Here's the drawing with two shaded views (mm, measured from the low corner). I have some questions. A direction names the side the tool comes from. Round coordinates to 2 decimals unless told otherwise and drop trailing zeros. Order: outer loops, then holes, each group sorted by start corner. A loop starts at its lowest first (then second) coordinate and runs counter-clockwise, first axis right, second up. Notation, with made-up numbers: (82, 20) -> (97, 20) arc R23 cw to (97, 35) -> close; hole circle Ø8 at (-25, 68). An arc over 180 degrees is marked (long way). Answer in a Markdown table with one row per item.
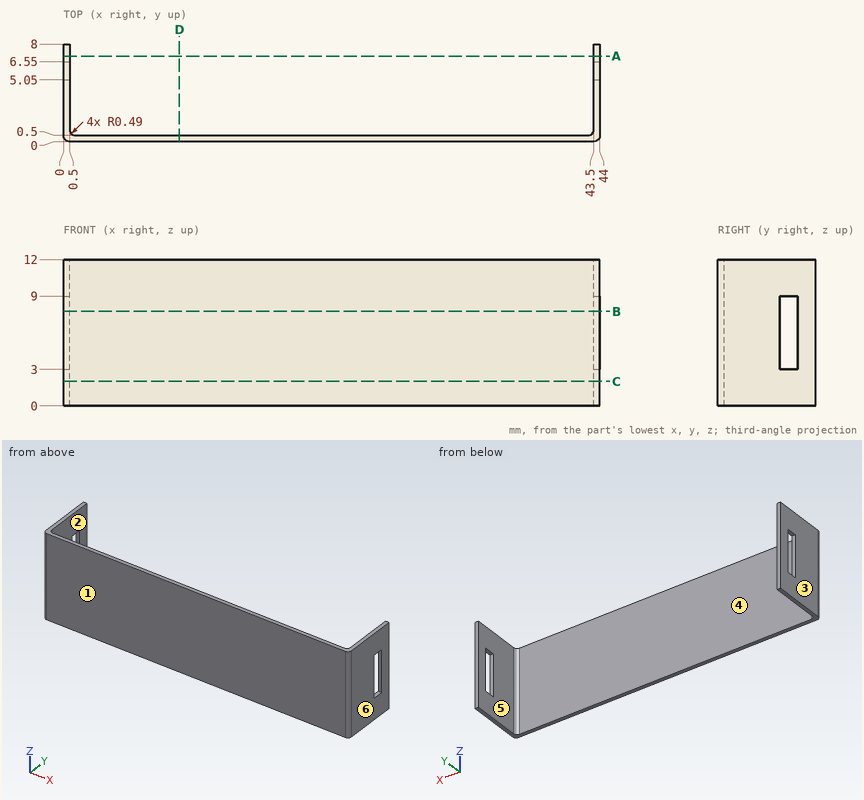
1. Suppose I cut it at B-B on z = 7.75. Write out the boundary of the cut face in (x, y), then the cut area to 3 significant figures.
Numbers:
| item | result |
|---|---|
| outline | (0, 0.49) arc R0.49 ccw to (0.49, 0) -> (43.51, 0) arc R0.49 ccw to (44, 0.49) -> (44, 5.05) -> (43.5, 5.05) -> (43.5, 0.99) arc R0.49 cw to (43.01, 0.5) -> (0.99, 0.5) arc R0.49 cw to (0.5, 0.99) -> (0.5, 5.05) -> (0, 5.05) -> close; (0, 6.55) -> (0.5, 6.55) -> (0.5, 8) -> (0, 8) -> close; (43.5, 6.55) -> (44, 6.55) -> (44, 8) -> (43.5, 8) -> close |
| area | 28.0 mm2 |
2. We'd pull the mould along X, two halves only. Please class the marked faces 1, 2, 3 and 4: released by +X, released by -X, zero draft, split by the parting line, or undercut.
Numbers:
| item | result |
|---|---|
| face 1 | zero draft |
| face 2 | undercut |
| face 3 | released by -X |
| face 4 | undercut |
3. For the marked faces 5 and 6, which set-ups out of +Z, -Z, +X, -X, +Y, -Y let a thin tool reach every point of the face, with its end or its side?
Numbers:
| item | result |
|---|---|
| face 5 | +Z, -Z, +Y |
| face 6 | +Z, -Z, +X, +Y, -Y |
4. Suppose I cut it at A-A on y = 7. Write out the boundary of the cut face in (x, z).
Numbers:
| item | result |
|---|---|
| outline | (0, 0) -> (0.5, 0) -> (0.5, 12) -> (0, 12) -> close; (43.5, 0) -> (44, 0) -> (44, 12) -> (43.5, 12) -> close |
5. Please list where these lines run through material, in increasing order: line 1 along X through (y, z) = (2.25, 8.75); line 2 along Y through (x, z) = (13, 0.5).
Numbers:
| item | result |
|---|---|
| line 1 | x = 0 to 0.5, 43.5 to 44 |
| line 2 | y = 0 to 0.5 |
6. For pin 1 Ø1.5 at (y, z) = (1.5, 8.5) entering from -X; pin 2 Ø0.6 at (x, z) = (0, 6) entering from -Y, each with a flat end and sliding along its axis, tell me the tip position at first contact or that it passes through.
Numbers:
| item | result |
|---|---|
| pin 1 | stops at x = 0 |
| pin 2 | stops at y = 0.04 |
7. Suppose I cut it at D-D on x = 9.5. Write out the boundary of the cut face in (y, z), then the cut area to 3 significant figures.
Numbers:
| item | result |
|---|---|
| outline | (0, 0) -> (0.5, 0) -> (0.5, 12) -> (0, 12) -> close |
| area | 6.00 mm2 |
8. Suppose I cut it at C-C on z = 2. Write out the boundary of the cut face in (x, y).
Numbers:
| item | result |
|---|---|
| outline | (0, 0.49) arc R0.49 ccw to (0.49, 0) -> (43.51, 0) arc R0.49 ccw to (44, 0.49) -> (44, 8) -> (43.5, 8) -> (43.5, 0.99) arc R0.49 cw to (43.01, 0.5) -> (0.99, 0.5) arc R0.49 cw to (0.5, 0.99) -> (0.5, 8) -> (0, 8) -> close |
